from build123d import *

# Parameters (mm, degrees)
CROQUIS1_W               = 28.575
CROQUIS1_H               = 50.8
BRIDA_BASE1_DEPTH        = 1.524
CROQUIS6_R               = 3.9751
CROQUIS6_W               = 3.1115
CROQUIS6_H               = 21.59
CROQUIS6_H_2             = 12.7
CORTAR_EXTRUIR1_DEPTH    = 30.182447331
BRIDA_START              = -12.7
BRIDA_DE_ARISTA1_DEPTH   = 16.51
BRIDA_START_2            = -12.8524
BRIDA_DE_ARISTA1_2_DEPTH = 0.1524
BRIDA_START_3            = 3.81
BRIDA_DE_ARISTA1_3_DEPTH = 0.1524
BRIDA_DE_ARISTA1_4_DEPTH = 16.51
CROQUIS13_W              = 1.524
CROQUIS13_H              = 4.826
SALIENTE_EXTRUIR1_DEPTH  = 21.59
REDONDEO1_R              = 3.302
REDONDEO2_R              = 1.524


# Read off the part's stored shape, not the designer's step: Brida de arista1
# Sheet-metal steps are written as plain solids
with BuildPart() as part:
    # Croquis1 → Brida base1 (new body)
    with BuildSketch(Plane.XY):
        Rectangle(CROQUIS1_W, CROQUIS1_H)
    extrude(amount=-BRIDA_BASE1_DEPTH)

    # Croquis6 → Cortar-Extruir1 (cut, through all)
    with BuildSketch(Plane.XY):
        with Locations((0, -12.7)):
            Circle(CROQUIS6_R)
        with Locations((-12.73175, 14.605)):
            Rectangle(CROQUIS6_W, CROQUIS6_H)
        with Locations((12.73175, 14.605)):
            Rectangle(CROQUIS6_W, CROQUIS6_H)
        with Locations((-12.73175, -19.05)):
            Rectangle(CROQUIS6_W, CROQUIS6_H_2)
        with Locations((12.73175, -19.05)):
            Rectangle(CROQUIS6_W, CROQUIS6_H_2)
    extrude(amount=-CORTAR_EXTRUIR1_DEPTH, mode=Mode.SUBTRACT)

    # Brida de arista1 outline → Brida de arista1 (cut)
    with BuildSketch(Plane(origin=(0, 0, 0), x_dir=(1, 0, 0), z_dir=(0, 1, 0)).offset(BRIDA_START)):
        with BuildLine():
            Line((14.2875, 1.524), (11.2395, 1.524))
            ThreePointArc((11.2395, 1.524), (12.7635, 1.115645431), (13.879145431, 0))
            Line((13.879145431, 0), (14.2875, 0))
            Line((14.2875, 0), (14.2875, 1.524))
        make_face()
        with BuildLine():
            ThreePointArc((-13.879145431, 0), (-12.7635, 1.115645431), (-11.2395, 1.524))
            Line((-11.2395, 1.524), (-14.2875, 1.524))
            Line((-14.2875, 1.524), (-14.2875, 0))
            Line((-14.2875, 0), (-13.879145431, 0))
        make_face()
    extrude(amount=BRIDA_DE_ARISTA1_DEPTH, mode=Mode.SUBTRACT)

    # Brida de arista1 2 outline → Brida de arista1 2 (cut)
    with BuildSketch(Plane(origin=(0, 0, 0), x_dir=(1, 0, 0), z_dir=(0, 1, 0)).offset(BRIDA_START_2)):
        with BuildLine():
            Line((11.0871, 1.524), (11.0871, 0))
            Line((11.0871, 0), (13.879145431, 0))
            ThreePointArc((13.879145431, 0), (12.7635, 1.115645431), (11.2395, 1.524))
            Line((11.2395, 1.524), (11.0871, 1.524))
        make_face()
        with BuildLine():
            Line((-13.879145431, 0), (-11.0871, 0))
            Line((-11.0871, 0), (-11.0871, 1.524))
            Line((-11.0871, 1.524), (-11.2395, 1.524))
            ThreePointArc((-11.2395, 1.524), (-12.7635, 1.115645431), (-13.879145431, 0))
        make_face()
    extrude(amount=BRIDA_DE_ARISTA1_2_DEPTH, mode=Mode.SUBTRACT)

    # Brida de arista1 3 outline → Brida de arista1 3 (cut)
    with BuildSketch(Plane(origin=(0, 0, 0), x_dir=(1, 0, 0), z_dir=(0, 1, 0)).offset(BRIDA_START_3)):
        with BuildLine():
            Line((11.0871, 1.524), (11.0871, 0))
            Line((11.0871, 0), (13.879145431, 0))
            ThreePointArc((13.879145431, 0), (12.7635, 1.115645431), (11.2395, 1.524))
            Line((11.2395, 1.524), (11.0871, 1.524))
        make_face()
        with BuildLine():
            Line((-13.879145431, 0), (-11.0871, 0))
            Line((-11.0871, 0), (-11.0871, 1.524))
            Line((-11.0871, 1.524), (-11.2395, 1.524))
            ThreePointArc((-11.2395, 1.524), (-12.7635, 1.115645431), (-13.879145431, 0))
        make_face()
    extrude(amount=BRIDA_DE_ARISTA1_3_DEPTH, mode=Mode.SUBTRACT)

    # Brida de arista1 4 outline → Brida de arista1 4 (add)
    with BuildSketch(Plane(origin=(0, 0, 0), x_dir=(1, 0, 0), z_dir=(0, 1, 0)).offset(BRIDA_START)):
        with BuildLine():
            Line((13.879145431, 0), (11.2395, 0))
            ThreePointArc((11.2395, 0), (12.317130735, -0.446369265), (12.7635, -1.524))
            Line((12.7635, -1.524), (12.7635, -18.288))
            Line((12.7635, -18.288), (14.2875, -18.288))
            Line((14.2875, -18.288), (14.2875, -1.524))
            ThreePointArc((14.2875, -1.524), (14.183641918, -0.735119551), (13.879145431, 0))
        make_face()
        with BuildLine():
            ThreePointArc((-12.7635, -1.524), (-12.317130735, -0.446369265), (-11.2395, 0))
            Line((-11.2395, 0), (-13.879145431, 0))
            ThreePointArc((-13.879145431, 0), (-14.183641918, -0.735119551), (-14.2875, -1.524))
            Line((-14.2875, -1.524), (-14.2875, -18.288))
            Line((-14.2875, -18.288), (-12.7635, -18.288))
            Line((-12.7635, -18.288), (-12.7635, -1.524))
        make_face()
    extrude(amount=BRIDA_DE_ARISTA1_4_DEPTH)

    # Croquis13 → Saliente-Extruir1 (add)
    with BuildSketch(Plane(origin=(0, 3.81, 0), x_dir=(1, 0, 0), z_dir=(0, 1, 0))):
        with Locations((13.5255, -15.875)):
            Rectangle(CROQUIS13_W, CROQUIS13_H)
    saliente_extruir1 = extrude(amount=SALIENTE_EXTRUIR1_DEPTH)

    # Simetría1: Saliente-Extruir1 across plane
    add(saliente_extruir1.mirror(Plane(origin=(0, 0, 0), x_dir=(0, 0, 1), z_dir=(1, 0, 0))))

    # Redondeo1
    redondeo1_edges = [part.edges().sort_by_distance(p)[0] for p in [
        (11.176, 25.4, -0.762),
        (-11.176, -25.4, -0.762),
        (11.176, -25.4, -0.762),
        (-11.176, 25.4, -0.762),
    ]]
    fillet(redondeo1_edges, radius=REDONDEO1_R)

    # Redondeo2
    redondeo2_edges = [part.edges().sort_by_distance(p)[0] for p in [
        (13.5255, -12.7, 18.288),
        (-13.5255, -12.7, 18.288),
        (13.5255, 25.4, 18.288),
        (13.5255, 25.4, 13.462),
        (-13.5255, 25.4, 13.462),
        (-13.5255, 25.4, 18.288),
    ]]
    fillet(redondeo2_edges, radius=REDONDEO2_R)


solid = part.part
Can you work these out from the model? Positions are in its coordinate system, mm. A direction names the side the tool comes from. Coordinates: 2 decimals unless noted, no trailing zeros. Write each loop counter-clockwise with the first axis right and the second up, starting at its lowest first coordinate (ties: lowest second). Pieces come first, ordered by that corner, then holes. Notation, with made-up numbers: (69.5, -15) - (82.5, -15) arc R19 ccw to (82.5, 20) - close; hole circle Ø4 at (-22.5, 3). An arc over 180 degrees is marked (long way). Return JSON: item names as keys, results as strings. Group by question number.
Item 1: I'm going to push flat-ended pins straight in: pin 1 Ø5 at (y, z) = (7, 7) entering from -X; pin 2 Ø0.5 at (y, z) = (10.5, -1) entering from +X; pin 3 Ø6 at (x, z) = (10.5, 2.5) entering from -Y (3 decimals); pin 4 Ø1.2 at (y, z) = (15, -0.5) entering from -X. Where does each tip first touch, or does it pass through?
Item 2: Which directions (+Z, -Z, +X, -X, +Y, -Y) give clear straight access to the entire face, cutting with the end or side of a thin tool? Please do faces 5 (the face through (-10.18, 24.46, -0.77)), 6 (the face through (-14, 14, 13.462)), 7 (the face through (11.176, 13, -1)).
Item 3: If we section it at C-C (z = 7.75): Write out the boundary of the cut face in (x, y), then the cut area to 3 significant figures.
Item 4: If we section it at D-D (y = 0): Write out the boundary of the cut face in (x, z), then the cut area to 3 significant figures.
Item 5: Please list where these lines run through material, in increasing order: probe 1 along Y at (x, z) = (0, -1.15); probe 2 along X at (y, z) = (0, 3.25); probe 3 along Z at (x, y) = (9.5, -23).
Item 6: We'd pull the mould along X, two halves only. Please class faces 1 (the face through (-14.288, 2, 12)), 2 (the face through (-12.33, -4.56, 0.46)), 3 (the face through (-14, 25.4, 16)), 4 (the face through (-3.155, -15.119, -0.751)): pulls with the +X half, pulls with the -X half, needs draft (parallel to the pull), parting line crosses it, or undercut.
Item 7: If we section it at A-A (x = 0): Write out the boundary of the cut face in (y, z).
Item 8: If we section it at B-B (y = 13.5): Write out the boundary of the cut face in (x, z).
Return value:
{
 "1": {"pin 1": "passes through", "pin 2": "stops at x = 11.18", "pin 3": "stops at y = -25.255", "pin 4": "stops at x = -11.18"},
 "2": {"face 5": "+Z, -Z, -X, +Y", "face 6": "-Z, +X, -X, +Y", "face 7": "+Z, -Z, +X, +Y"},
 "3": {"outline": "(-14.29, -12.7) - (-12.76, -12.7) - (-12.76, 3.81) - (-14.29, 3.81) - close; (12.76, -12.7) - (14.29, -12.7) - (14.29, 3.81) - (12.76, 3.81) - close", "area": "50.3 mm^2"},
 "4": {"outline": "(-14.29, 1.52) arc R3.05 ccw to (-11.24, -1.52) - (11.24, -1.52) arc R3.05 ccw to (14.29, 1.52) - (14.29, 18.29) - (12.76, 18.29) - (12.76, 1.52) arc R1.52 cw to (11.24, 0) - (-11.24, 0) arc R1.52 cw to (-12.76, 1.52) - (-12.76, 18.29) - (-14.29, 18.29) - close", "area": "96.3 mm^2"},
 "5": {"probe 1": "y = -25.4 to -16.68, -8.72 to 25.4", "probe 2": "x = -14.29 to -12.76, 12.76 to 14.29", "probe 3": "z = -1.52 to 0"},
 "6": {"face 1": "pulls with the -X half", "face 2": "undercut", "face 3": "needs draft", "face 4": "undercut"},
 "7": {"outline": "(-25.4, -1.52) - (-16.68, -1.52) - (-16.68, 0) - (-25.4, 0) - close; (-8.72, -1.52) - (25.4, -1.52) - (25.4, 0) - (-8.72, 0) - close"},
 "8": {"outline": "(-14.29, 13.46) - (-12.76, 13.46) - (-12.76, 18.29) - (-14.29, 18.29) - close; (-11.18, -1.52) - (11.18, -1.52) - (11.18, 0) - (-11.18, 0) - close; (12.76, 13.46) - (14.29, 13.46) - (14.29, 18.29) - (12.76, 18.29) - close"}
}
